Could you check a few things on this model? Use its own coordinates, in mm. A direction names the side the tool comes from. Coordinates: 2 decimals unless noted, no trailing zeros. Loops run counter-clockwise (first coordinate to the right, second up) from the corner with the lowest first, then second, coordinate; pieces in that order, holes last. Notation, with made-up numbers: (-23.75, 64.5) -> (-13.75, 64.5) arc R21 ccw to (-13.75, 78.5) -> close; hole circle Ø1 at (72, -6). An arc over 180 degrees is marked (long way). One line per question, with ' | ' between items.
Autodesk Inventor part; units mm, degrees
ref_plane "YZ Plane" through (0, 0, 0) normal (1, 0, 0) x (0, 1, 0)
ref_plane "XZ Plane" through (0, 0, 0) normal (0, 1, 0) x (-1, 0, 0)
ref_plane "XY Plane" through (0, 0, 0) normal (0, 0, 1) x (1, 0, 0)
sketch "Sketch1" plane through (0, 0, 0) normal (0, 0, 1) x (1, 0, 0)
  circle A0 centre (0, 0) radius 7
  dimension "d0" = 14
extrude "Extrusion1" add sketch "Sketch1" along normal blind 12
sketch "Sketch2" plane through (0, 0, 12) normal (0, 0, 1) x (1, 0, 0)
  circle A0 centre (0, 0) radius 10
  dimension "d3" = 20
extrude "Extrusion2" add sketch "Sketch2" along normal blind 8
sketch "Sketch3" plane through (0, 0, 20) normal (0, 0, 1) x (1, 0, 0)
  circle A0 centre (0, 0) radius 10.9378
extrude "Extrusion3" add sketch "Sketch3" along normal blind 14
sketch "Sketch4" plane through (0, 0, 34) normal (0, 0, 1) x (1, 0, 0)
  circle A0 centre (0, 0) radius 10
extrude "Extrusion4" add sketch "Sketch4" along normal blind 9
sketch "Sketch5" plane through (0, 0, 43) normal (0, 0, 1) x (1, 0, 0)
  circle A0 centre (0, 0) radius 7
  dimension "d10" = 14
extrude "Extrusion5" add sketch "Sketch5" along normal blind 12
properties part number "eje escalonado"
1) If we section it at D-D on y = 8.75: Please give me the cut outline in (x, z).
Data:
outline: (-6.56, 20) -> (-4.84, 20) -> (-4.84, 12) -> (4.84, 12) -> (4.84, 20) -> (6.56, 20) -> (6.56, 34) -> (4.84, 34) -> (4.84, 43) -> (-4.84, 43) -> (-4.84, 34) -> (-6.56, 34) -> close
2) I'm going to push flat-ended pins straight in: pin 1 Ø5 at (y, z) = (-3.5, 32.5) entering from +X; pin 2 Ø12 at (y, z) = (8.5, 28) entering from +X. Where does each tip first touch, or does it pass through?
Data:
pin 1: x = 10.89 | pin 2: x = 10.65
3) If we section it at A-A on x = 0: Please give me the cut outline in (y, z).
Data:
outline: (-10.94, 20) -> (-10, 20) -> (-10, 12) -> (-7, 12) -> (-7, 0) -> (7, 0) -> (7, 12) -> (10, 12) -> (10, 20) -> (10.94, 20) -> (10.94, 34) -> (10, 34) -> (10, 43) -> (7, 43) -> (7, 55) -> (-7, 55) -> (-7, 43) -> (-10, 43) -> (-10, 34) -> (-10.94, 34) -> close
4) If we section it at C-C on z = 10: Please give me the cut outline in (x, y), and give its area (3 significant figures).
Data:
outline: circle Ø14 at (0, 0) | area: 154 mm²
5) On a 3-axis mill with a long thin cutter (end or side, diameter ignored), from which of +Z, -Z, +X, -X, +Y, -Y can I reach the whole of each face in a straight line? I mean faces 1 (the face through (6.466, 2.681, 5.916)), 2 (the face through (6.466, 2.681, 48.916)), 3 (the face through (-1.424, -10.845, 26.902)). Say none if no direction works.
Data:
face 1: -Z | face 2: +Z | face 3: +Z, -Z
6) I need wall thicknesses on line 1 along Z through (x, y) = (-5.5, 4.75); line 2 along Z through (x, y) = (-9.25, -4.75); line 3 along Y through (x, z) = (-6, 52). Which ranges of each line are inside material? Lowest first, please. Write a range as from..to.
Data:
line 1: 12..43 | line 2: 20..34 | line 3: -3.61..3.61
